```python
from build123d import *

# Parameters (mm, degrees)
SKETCH_1_W          = 108
SKETCH_1_H          = 138
EXTRUDE_1_DEPTH     = 4
SKETCH_2_W          = 69.21
SKETCH_2_H          = 50.1
CUT_EXTRUDE_1_DEPTH = 176.282628917
SKETCH_4_W          = 15
SKETCH_4_H          = 4
EXTRUDE_2_DEPTH     = 6
SKETCH_6_W          = 9
SKETCH_6_H          = 4
EXTRUDE_3_DEPTH     = 6
SKETCH_7_W          = 15
SKETCH_7_H          = 4
EXTRUDE_4_DEPTH     = 6
SKETCH_8_W          = 9
SKETCH_8_H          = 4
EXTRUDE_5_DEPTH     = 6
SKETCH_9_W          = 10
SKETCH_9_H          = 4
EXTRUDE_6_DEPTH     = 6
SKETCH_10_W         = 10
SKETCH_10_H         = 4
EXTRUDE_7_DEPTH     = 6
SKETCH_11_W         = 11.5
SKETCH_11_H         = 11.8
SKETCH_11_W_2       = 11.8
CUT_EXTRUDE_2_DEPTH = 184.706287318
SKETCH_12_W         = 11.8
SKETCH_12_H         = 11.8
CUT_EXTRUDE_3_DEPTH = 184.706287318
SKETCH_13_W         = 11.8
SKETCH_13_H         = 11.8
CUT_EXTRUDE_4_DEPTH = 184.706287318
SKETCH_14_R         = 1.3
SKETCH_14_W         = 29.8
SKETCH_14_H         = 1.8
SKETCH_14_W_2       = 39.9
SKETCH_14_H_2       = 3.2
CUT_EXTRUDE_5_DEPTH = 184.706287318


with BuildPart() as part:
    # Эскиз1 → Бобышка-Вытянуть1 (new body)
    with BuildSketch(Plane(origin=(0, 0, 0), x_dir=(1, 0, 0), z_dir=(0, 1, 0))):
        with Locations((54, -69)):
            Rectangle(SKETCH_1_W, SKETCH_1_H)
    extrude(amount=EXTRUDE_1_DEPTH)

    # Эскиз2 → Вырез-Вытянуть1 (cut, through all)
    with BuildSketch(Plane(origin=(0, 4, 0), x_dir=(1, 0, 0), z_dir=(0, 1, 0))):
        with Locations((48.505, -35.05)):
            Rectangle(SKETCH_2_W, SKETCH_2_H)
    extrude(amount=-CUT_EXTRUDE_1_DEPTH, mode=Mode.SUBTRACT)

    # Эскиз4 → Бобышка-Вытянуть2 (add)
    with BuildSketch(Plane.ZY):
        with Locations((11.5, 2)):
            Rectangle(SKETCH_4_W, SKETCH_4_H)
        with Locations((36.5, 2)):
            Rectangle(SKETCH_4_W, SKETCH_4_H)
        with Locations((61.5, 2)):
            Rectangle(SKETCH_4_W, SKETCH_4_H)
        with Locations((86.5, 2)):
            Rectangle(SKETCH_4_W, SKETCH_4_H)
        with Locations((111.5, 2)):
            Rectangle(SKETCH_4_W, SKETCH_4_H)
    extrude(amount=EXTRUDE_2_DEPTH)

    # Эскиз6 → Бобышка-Вытянуть3 (add)
    with BuildSketch(Plane.ZY):
        with Locations((133.5, 2)):
            Rectangle(SKETCH_6_W, SKETCH_6_H)
    extrude(amount=EXTRUDE_3_DEPTH)

    # Эскиз7 → Бобышка-Вытянуть4 (add)
    with BuildSketch(Plane(origin=(108, 0, 0), x_dir=(0, 0, -1), z_dir=(1, 0, 0))):
        with Locations((-11.5, 2)):
            Rectangle(SKETCH_7_W, SKETCH_7_H)
        with Locations((-36.5, 2)):
            Rectangle(SKETCH_7_W, SKETCH_7_H)
        with Locations((-61.5, 2)):
            Rectangle(SKETCH_7_W, SKETCH_7_H)
        with Locations((-86.5, 2)):
            Rectangle(SKETCH_7_W, SKETCH_7_H)
        with Locations((-111.5, 2)):
            Rectangle(SKETCH_7_W, SKETCH_7_H)
    extrude(amount=EXTRUDE_4_DEPTH)

    # Эскиз8 → Бобышка-Вытянуть5 (add)
    with BuildSketch(Plane(origin=(108, 0, 0), x_dir=(0, 0, -1), z_dir=(1, 0, 0))):
        with Locations((-133.5, 2)):
            Rectangle(SKETCH_8_W, SKETCH_8_H)
    extrude(amount=EXTRUDE_5_DEPTH)

    # Эскиз9 → Бобышка-Вытянуть6 (add)
    with BuildSketch(Plane(origin=(0, 0, 0), x_dir=(-1, 0, 0), z_dir=(0, 0, -1))):
        with Locations((-94.998495411, 2)):
            Rectangle(SKETCH_9_W, SKETCH_9_H)
        with Locations((-74.998495411, 2)):
            Rectangle(SKETCH_9_W, SKETCH_9_H)
        with Locations((-54.998495411, 2)):
            Rectangle(SKETCH_9_W, SKETCH_9_H)
        with Locations((-34.998495411, 2)):
            Rectangle(SKETCH_9_W, SKETCH_9_H)
        with Locations((-14.998495411, 2)):
            Rectangle(SKETCH_9_W, SKETCH_9_H)
    extrude(amount=EXTRUDE_6_DEPTH)

    # Эскиз10 → Бобышка-Вытянуть7 (add)
    with BuildSketch(Plane.XY.offset(138)):
        with Locations((15, 2)):
            Rectangle(SKETCH_10_W, SKETCH_10_H)
        with Locations((35, 2)):
            Rectangle(SKETCH_10_W, SKETCH_10_H)
        with Locations((55, 2)):
            Rectangle(SKETCH_10_W, SKETCH_10_H)
        with Locations((75, 2)):
            Rectangle(SKETCH_10_W, SKETCH_10_H)
        with Locations((95, 2)):
            Rectangle(SKETCH_10_W, SKETCH_10_H)
    extrude(amount=EXTRUDE_7_DEPTH)

    # Эскиз11 → Вырез-Вытянуть2 (cut, through all)
    with BuildSketch(Plane(origin=(0, 4, 0), x_dir=(1, 0, 0), z_dir=(0, 1, 0))):
        with Locations((10.75, -90.1)):
            Rectangle(SKETCH_11_W, SKETCH_11_H)
        with Locations((10.9, -76.3)):
            Rectangle(SKETCH_11_W_2, SKETCH_11_H)
    extrude(amount=-CUT_EXTRUDE_2_DEPTH, mode=Mode.SUBTRACT)

    # Эскиз12 → Вырез-Вытянуть3 (cut, through all)
    with BuildSketch(Plane(origin=(0, 4, 0), x_dir=(1, 0, 0), z_dir=(0, 1, 0))):
        with Locations((83.3, -127.1)):
            Rectangle(SKETCH_12_W, SKETCH_12_H)
        with Locations((97.1, -127.1)):
            Rectangle(SKETCH_12_W, SKETCH_12_H)
    extrude(amount=-CUT_EXTRUDE_3_DEPTH, mode=Mode.SUBTRACT)

    # Эскиз13 → Вырез-Вытянуть4 (cut, through all)
    with BuildSketch(Plane(origin=(0, 4, 0), x_dir=(1, 0, 0), z_dir=(0, 1, 0))):
        with Locations((10.9, -127.1)):
            Rectangle(SKETCH_13_W, SKETCH_13_H)
    extrude(amount=-CUT_EXTRUDE_4_DEPTH, mode=Mode.SUBTRACT)

    # Эскиз14 → Вырез-Вытянуть5 (cut, through all)
    with BuildSketch(Plane(origin=(0, 4, 0), x_dir=(1, 0, 0), z_dir=(0, 1, 0))):
        with Locations(Location((38.25, -72.1, 0), (0, 0, 270))):
            Circle(SKETCH_14_R)
        with Locations(Location((69.75, -72.1, 0), (0, 0, 270))):
            Circle(SKETCH_14_R)
        with Locations((54, -67.1)):
            Rectangle(SKETCH_14_W, SKETCH_14_H)
        with Locations((54, -87.1)):
            Rectangle(SKETCH_14_W_2, SKETCH_14_H_2)
    extrude(amount=-CUT_EXTRUDE_5_DEPTH, mode=Mode.SUBTRACT)


solid = part.part
```
Input: part model. Units: mm. Frame: model coordinates. A direction names the side the tool comes from. Give positions to 0.01 mm unless a question says otherwise; leave off trailing zeros. Write each loop counter-clockwise with the first axis right and the second up, starting at its lowest first coordinate (ties: lowest second). Pieces come first, ordered by that corner, then holes. Notation, with made-up numbers: (45.5, 84) - (92.5, 84) arc R32 cw to (92.5, 113) - close; hole circle Ø8 at (22, 63.25). An arc over 180 degrees is marked (long way). Write item = value, one per line. Start each with the question number.
1. Ray query, L1, parallel to Z at x = 36.5, y = 3.3; L2, parallel to X at y = 1.7, z = 72.1; L3, parallel to X at y = 0.55, z = 127. Return the intervals inside material, ascending.
2. Access query for faces 5 (the flat face through (111, 2, 44)), 6 (the flat face through (80, 2, 141)), 7 (the flat face through (-3, 2, 4)), 8 (the flat face through (91.2, 2, 127)), 9 (the flat face through (-3, 2, 79)). Directions: +Z, -Z, +X, -X, +Y, -Y. A direction counts if a zero-diameter tool reaches every point of the face in a straight line with its end or side. Return the directions, or none.
3. First-contact query: pin 1 Ø1.2 at (x, y) = (83, 1.5) entering from -Z; pin 2 Ø1.2 at (x, y) = (112, 2.5) entering from +Z; pin 3 Ø2 at (y, z) = (2, 126) entering from -X. Flat tips, straight axial feed; report the tip coordinate or a pass-through.
4. Section query C-C, the plane x = 86. Output: boundary loops of the cut face in (y, z), then the cut area to 3 significant figures.
5. Mould query, pull axis X, two halves, no side actions, for faces 1 (the flat face through (53, 4, 70)), 2 (the flat face through (69.998, 2, -3)), 3 (the flat face through (0, 2, 124)), 4 (the flat face through (54, 2, 66.2)). Classes: released by +X, released by -X, zero draft, split by the parting line, or undercut.
6. Section query B-B, the plane z = 15.5. Output: boundary loops of the cut face in (x, y), then the cut area to 3 significant figures.
7. Section query A-A, the plane x = 63.5. Output: boundary loops of the cut face in (y, z).
Check sheet entries:
q1.L1 = -6 to 10, 60.1 to 85.5, 88.7 to 144
q1.L2 = 0 to 5, 16.8 to 36.95, 39.55 to 68.45, 71.05 to 108
q1.L3 = 0 to 5, 16.8 to 77.4, 89.2 to 91.2, 103 to 108
q2.face_5 = +X, +Y, -Y
q2.face_6 = +Z, +Y, -Y
q2.face_7 = -Z, -X, +Y, -Y
q2.face_8 = +Y, -Y
q2.face_9 = -X, +Y, -Y
q3.pin_1 = 0
q3.pin_2 = 138
q3.pin_3 = 0
q4.outline = (0, 0) - (4, 0) - (4, 121.2) - (0, 121.2) - close; (0, 133) - (4, 133) - (4, 138) - (0, 138) - close
q4.area = 505 mm2
q5.face_1 = zero draft
q5.face_2 = undercut
q5.face_3 = released by -X
q5.face_4 = undercut
q6.outline = (-6, 0) - (13.9, 0) - (13.9, 4) - (-6, 4) - close; (83.11, 0) - (114, 0) - (114, 4) - (83.11, 4) - close
q6.area = 203 mm2
q7.outline = (0, 0) - (4, 0) - (4, 10) - (0, 10) - close; (0, 60.1) - (4, 60.1) - (4, 66.2) - (0, 66.2) - close; (0, 68) - (4, 68) - (4, 85.5) - (0, 85.5) - close; (0, 88.7) - (4, 88.7) - (4, 138) - (0, 138) - close
